Design review of the part built by this model. Coordinates are the model's own, in mm. Face numbers are marked on the shaded views. Give positions to 0.01 mm unless a question says otherwise; leave off trailing zeros. Order: outer loops, then holes, each group sorted by start corner. A loop starts at its lowest first (then second) coordinate and runs counter-clockwise, first axis right, second up. Notation, with made-up numbers: (63, -38.75) - (74, -38.75) arc R21 cw to (74, -22.75) - close; hole circle Ø8 at (70.25, 51). An arc over 180 degrees is marked (long way). Write each question's results on one line, items separated by ' | '. Start each with the question number.
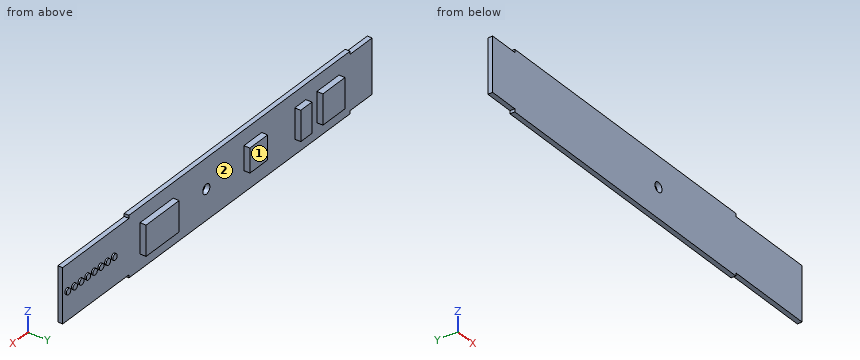
Autodesk Inventor part; units mm, degrees
ref_plane "YZ Plane" through (0, 0, 0) normal (1, 0, 0) x (0, 1, 0)
ref_plane "XZ Plane" through (0, 0, 0) normal (0, 1, 0) x (-1, 0, 0)
ref_plane "XY Plane" through (0, 0, 0) normal (0, 0, 1) x (1, 0, 0)
sketch "草图1" plane through (0, 0, 0) normal (0, 1, 0) x (-1, 0, 0)
  line L0 (0, 20) -> (-100, 20)
  line L1 (-100, 20) -> (-100, 0)
  line L2 (-100, 0) -> (0, 0)
  line L3 (0, 0) -> (0, 20)
  point P0 (0, 0)
  dimension "d0" = 20
  dimension "d1" = 100
extrude "拉伸1" add sketch "草图1" along normal blind 1.6
sketch "草图2" plane through (0, 1.6, 0) normal (0, 1, 0) x (1, 0, 0)
  line L0 (5, -15) -> (15, -15)
  line L1 (15, -15) -> (15, -5)
  line L2 (15, -5) -> (5, -5)
  line L3 (5, -5) -> (5, -15)
  line L4 (100, 0) -> (0, 0)
  line L5 (0, 0) -> (0, -20)
  point P0 (0, 0)
  dimension "d4" = 10
  dimension "d5" = 10
  dimension "d6" = 5
  dimension "d7" = 5
extrude "拉伸2" add sketch "草图2" along normal blind 2
sketch "草图3" plane through (0, 1.6, 0) normal (0, 1, 0) x (1, 0, 0)
  line L0 (80, -15) -> (95, -15)
  line L1 (95, -15) -> (95, -5)
  line L2 (95, -5) -> (80, -5)
  line L3 (80, -5) -> (80, -15)
  line L4 (100, 0) -> (0, 0)
  line L5 (100, -20) -> (100, 0)
  point P0 (0, 0)
  point P1 (100, -10)
  point P2 (95, -10)
  dimension "d10" = 10
  dimension "d11" = 15
  dimension "d12" = 5
  dimension "d13" = 5
extrude "拉伸3" add sketch "草图3" along normal blind 2
sketch "草图4" plane through (0, 1.6, 0) normal (0, 1, 0) x (1, 0, 0)
  line L0 (48, -15) -> (40, -15)
  line L1 (40, -15) -> (40, -7)
  line L2 (40, -7) -> (48, -7)
  line L3 (48, -7) -> (48, -15)
  line L4 (0, -20) -> (100, -20)
  line L5 (0, 0) -> (0, -20)
  point P0 (0, 0)
  point P1 (44, -15)
  dimension "d16" = 8
  dimension "d17" = 8
  dimension "d18" = 5
  dimension "d19" = 40
extrude "拉伸4" add sketch "草图4" along normal blind 2
sketch "草图5" plane through (0, 1.6, 0) normal (0, 1, 0) x (1, 0, 0)
  line L0 (25, -15) -> (20, -15)
  line L1 (20, -15) -> (20, -5)
  line L2 (20, -5) -> (25, -5)
  line L3 (25, -5) -> (25, -15)
  line L4 (0, -20) -> (100, -20)
  line L5 (0, 0) -> (0, -20)
  point P0 (0, 0)
  point P1 (20, -10)
  dimension "d22" = 5
  dimension "d23" = 10
  dimension "d24" = 5
  dimension "d25" = 20
extrude "拉伸5" add sketch "草图5" along normal blind 2
sketch "草图6" plane through (100, 0, 20) normal (1, 0, 0) x (0, 0, -1)
  point P0 (20, 0)
sketch "草图7" plane through (100, 0, 20) normal (1, 0, 0) x (0, 0, -1)
  line L0 (1, 0) -> (19, 0)
  line L1 (19, 0) -> (19, 1.6)
  line L2 (19, 1.6) -> (1, 1.6)
  line L3 (1, 1.6) -> (1, 0)
  line L4 (0, 0) -> (20, 0)
  line L5 (20, 0) -> (20, 1.6)
  point P0 (20, 0)
  point P1 (20, 0.8)
  dimension "d28" = 1.6
  dimension "d29" = 0
  dimension "d30" = 18
  dimension "d31" = 1
extrude "拉伸6" add sketch "草图7" along normal blind 30
sketch "草图8" plane through (0, 0, 0) normal (-1, 0, 0) x (0, 0, 1)
  line L0 (1, 1.6) -> (19, 1.6)
  line L1 (19, 1.6) -> (19, 0)
  line L2 (19, 0) -> (1, 0)
  line L3 (1, 0) -> (1, 1.6)
  line L4 (0, 0) -> (20, 0)
  line L5 (20, 0) -> (20, 1.6)
  point P0 (0, 0)
  dimension "d34" = 1.6
  dimension "d35" = 0
  dimension "d36" = 18
  dimension "d37" = 1
extrude "拉伸7" add sketch "草图8" along normal blind 10
sketch "草图9" plane through (0, 1.6, 0) normal (0, 1, 0) x (1, 0, 0)
  circle A0 centre (128, -10.5) radius 1
  line L0 (100, -1) -> (130, -1)
  line L1 (130, -1) -> (130, -19)
  circle A1 centre (125, -10.5) radius 1
  circle A2 centre (122, -10.5) radius 1
  circle A3 centre (119, -10.5) radius 1
  circle A4 centre (116, -10.5) radius 1
  circle A5 centre (113, -10.5) radius 1
  circle A6 centre (110, -10.5) radius 1
  circle A7 centre (107, -10.5) radius 1
  point P0 (0, 0)
  dimension "d40" = 2
  dimension "d41" = 9.5
  dimension "d42" = 2
  dimension "d45" = 3
extrude "拉伸8" add sketch "草图9" along normal blind 0.5
sketch "草图10" plane through (0, 1.6, 0) normal (0, 1, 0) x (1, 0, 0)
  circle A0 centre (65, -10) radius 1.6
  line L0 (100, 0) -> (0, 0)
  line L1 (0, 0) -> (0, -1)
  point P0 (0, -0.5)
  dimension "d52" = 3.2
  dimension "d53" = 10
  dimension "d54" = 65
extrude "拉伸9" cut sketch "草图10" against normal blind 1.6
properties part number "pcb板"
Q1. Add section B-B (y = 0.65). Give the boundary of the cut face in (x, z).
Q2. Insertion check: pin 1 Ø2 at (x, z) = (119, 11) entering from +Y; pin 2 Ø0.6 at (y, z) = (3, 10) entering from +X; pin 3 Ø2 at (x, y) = (104.5, 0.5) entering from -Z. Each pin has a flat end and moves straight along its axis. Give the tip position at first contact, or say it passes through.
Q3. Add section D-D (x = 28.5). Give the boundary of the cut face in (y, z).
Q4. Add section A-A (x = 65). Give the boundary of the cut face in (y, z), plus the area to 3 significant figures.
Q5. Add section C-C (x = 92). Give the boundary of the cut face in (y, z), plus the area to 3 significant figures.
Q6. Draft analysis for pull direction X (two halves, no side actions). For the marked faces 1 and 2, state which applies: pulls with the +X half, pulls with the -X half, needs draft (parallel to the pull), parting line crosses it, or undercut.
Q7. For line 1 (X direction, y = 3.1, z = 14); line 2 (Z direction, x = 65, y = 1); line 3 (X direction, y = 1.1, z = 10), list the stretches that pass through material, from the lowest coordinate up. Write a range as [from, to].
Verdict:
1) outline: (-10, 1) - (0, 1) - (0, 0) - (100, 0) - (100, 1) - (130, 1) - (130, 19) - (100, 19) - (100, 20) - (0, 20) - (0, 19) - (-10, 19) - close; hole circle Ø3.2 at (65, 10)
2) pin 1: stops at y = 2.1 | pin 2: stops at x = 95 | pin 3: stops at z = 1
3) outline: (0, 0) - (1.6, 0) - (1.6, 20) - (0, 20) - close
4) outline: (0, 0) - (1.6, 0) - (1.6, 8.4) - (0, 8.4) - close; (0, 11.6) - (1.6, 11.6) - (1.6, 20) - (0, 20) - close | area: 26.9 mm2
5) outline: (0, 0) - (1.6, 0) - (1.6, 5) - (3.6, 5) - (3.6, 15) - (1.6, 15) - (1.6, 20) - (0, 20) - close | area: 52.0 mm2
6) face 1: needs draft | face 2: undercut
7) line 1: x = [5, 15], [20, 25], [40, 48], [80, 95] | line 2: z = [0, 8.4], [11.6, 20] | line 3: x = [-10, 63.4], [66.6, 130]
